For this review, take the finished solid that the model builds, in its own axes (mm). A direction names the side the tool comes from. Give positions to 0.01 mm unless a question says otherwise; leave off trailing zeros. Order: outer loops, then holes, each group sorted by start corner. A loop starts at its lowest first (then second) coordinate and runs counter-clockwise, first axis right, second up. Notation, with made-up numbers: (-33, 77) - (-26, 77) arc R17 cw to (-26, 100) - close; hole circle Ø10 at (5, 27). An arc over 180 degrees is marked (long way). One line per item, written item: value.
```python
from build123d import *

# Parameters (mm, degrees)
BOSS_EXTRU_1_DEPTH                                 = 15
FRAISAGE_POUR_VIS_T_TE_FRAIS_E_CRUCIFO_D           = 3.2
FRAISAGE_POUR_VIS_T_TE_FRAIS_E_CRUCIFO_CSINK_D     = 6
FRAISAGE_POUR_VIS_T_TE_FRAIS_E_CRUCIFO_CSINK_ANGLE = 92
CONG_1_R                                           = 7


with BuildPart() as part:
    # Esquisse1 → Boss.-Extru.1 (new body)
    with BuildSketch(Plane.XY):
        Polygon((0, 13), (-40, 13), (-40, 8), (-25, 8), (-25, 0), (0, 0), align=None)
        Polygon((40, 13), (0, 13), (0, 0), (25, 0), (25, 8), (40, 8), align=None)
    extrude(amount=BOSS_EXTRU_1_DEPTH)

    # Fraisage pour vis à tête fraisée cruciforme M31 (through all)
    with Locations(Plane(origin=(0, 13, 0), x_dir=(1, 0, 0), z_dir=(0, 1, 0))):
        with Locations((-30, -7.5), (30, -7.5)):
            CounterSinkHole(FRAISAGE_POUR_VIS_T_TE_FRAIS_E_CRUCIFO_D / 2, FRAISAGE_POUR_VIS_T_TE_FRAIS_E_CRUCIFO_CSINK_D / 2, counter_sink_angle=FRAISAGE_POUR_VIS_T_TE_FRAIS_E_CRUCIFO_CSINK_ANGLE)

    # Congé1
    cong_1_edges = [part.edges().sort_by_distance(p)[0] for p in [
        (40, 10.5, 0),
        (25, 4, 0),
        (0, 0, 0),
        (-25, 0, 7.5),
        (25, 0, 7.5),
        (40, 10.5, 15),
        (-40, 10.5, 15),
        (-25, 4, 15),
        (0, 0, 15),
        (-25, 4, 0),
        (25, 4, 15),
        (-40, 10.5, 0),
    ]]
    fillet(cong_1_edges, radius=CONG_1_R)


solid = part.part
```
(1) Wall thickness on line 1 (X direction, y = 9.1, z = 7.5); line 2 (Z direction, x = -30, y = 9.1); line 3 (X direction, y = 10.75, z = 8.75): over which ranges is each line inside the solid? List them lowest first. Write a range as from..to.
Answers below:
line 1: x = -40..-31.6, -28.4..28.4, 31.6..40
line 2: z = 0..5.9, 9.1..15
line 3: x = -39.96..-31, -29..29, 31..39.96
(2) Machinability: for faces 1 (the face through (-23, 7.5, 2.1)), 2 (the face through (23, 7.5, 2.1)), 3 (the face through (22.9, 7.5, 13)), 4 (the face through (-22.9, 7.5, 13)), which of the approach directions +Z, -Z, +X, -X, +Y, -Y give a long, thin tool a straight path to every point of the face, cutting with its end or side? Answer none if there is none.
Answers below:
face 1: -Z, -X, -Y
face 2: -Z, +X, -Y
face 3: +Z, +X, -Y
face 4: +Z, -X, -Y
(3) Take a section at B-B (y = 1.75). Write out the cut boundary in (x, z).
Answers below:
outline: (-22.63, 7) arc R4.63 ccw to (-18, 2.37) - (18, 2.37) arc R4.63 ccw to (22.63, 7) - (22.63, 8) arc R4.63 ccw to (18, 12.63) - (-18, 12.63) arc R4.63 ccw to (-22.63, 8) - close
(4) Draft analysis for pull direction X (two halves, no side actions). For faces 5 (the face through (-28.73, 9.8, 8.47)), 6 (the face through (-22.9, 2, 7.5)), 7 (the face through (-32, 8, 7)), state which applies: pulls with the +X half, pulls with the -X half, needs draft (parallel to the pull), parting line crosses it, or undercut.
Answers below:
face 5: undercut
face 6: pulls with the -X half
face 7: needs draft
(5) For P1, Ø1.5, axis at y = 8.5, z = 11.5, coming from the -X side; P2, Ø4, axis at y = 5, z = 5, coming from the +X side; P3, Ø5, axis at x = 30, z = 7.5, coming from the +Y side; P4, Ø6, axis at y = 11, z = 9.5, coming from the +X side, all flat-tipped, find the tip position at first contact; note any pin that passes through.
Answers below:
P1: stops at x = -39.44
P2: stops at x = 24.95
P3: stops at y = 12.52
P4: stops at x = 40
(6) Take a section at C-C (z = 12.25). Write out the cut boundary in (x, y).
Answers below:
outline: (-38.56, 8) - (-23.56, 8) - (-23.56, 7) arc R5.56 ccw to (-18, 1.44) - (18, 1.44) arc R5.56 ccw to (23.56, 7) - (23.56, 8) - (38.56, 8) - (38.56, 13) - (-38.56, 13) - close
(7) Take a section at D-D (x = -19.5). Write out the cut boundary in (y, z).
Answers below:
outline: (0.16, 7) arc R6.84 ccw to (7, 0.16) - (8, 0.16) - (8, 0) - (13, 0) - (13, 15) - (8, 15) - (8, 14.84) - (7, 14.84) arc R6.84 ccw to (0.16, 8) - close
(8) Take a section at A-A (x = 30). Write out the cut boundary in (y, z).
Answers below:
outline: (8, 0) - (13, 0) - (13, 4.5) - (11.65, 5.9) - (8, 5.9) - close; (8, 9.1) - (11.65, 9.1) - (13, 10.5) - (13, 15) - (8, 15) - close
